Could you check a few things on this drawing? It's one solid part, dimensions in mm from its lowest x, y, z. A direction names the side the tool comes from. Give positions to 0.01 mm unless a question says otherwise; leave off trailing zeros. Loops run counter-clockwise (first coordinate to the right, second up) from the corner with the lowest first, then second, coordinate; pieces in that order, holes last. Notation, with made-up numbers: (85, 32.5) - (140, 32.5) arc R24 cw to (140, 58.5) - close; hole circle Ø6 at (74, 83). An arc over 180 degrees is marked (long way). Answer as a JSON object with one key per item and string values.
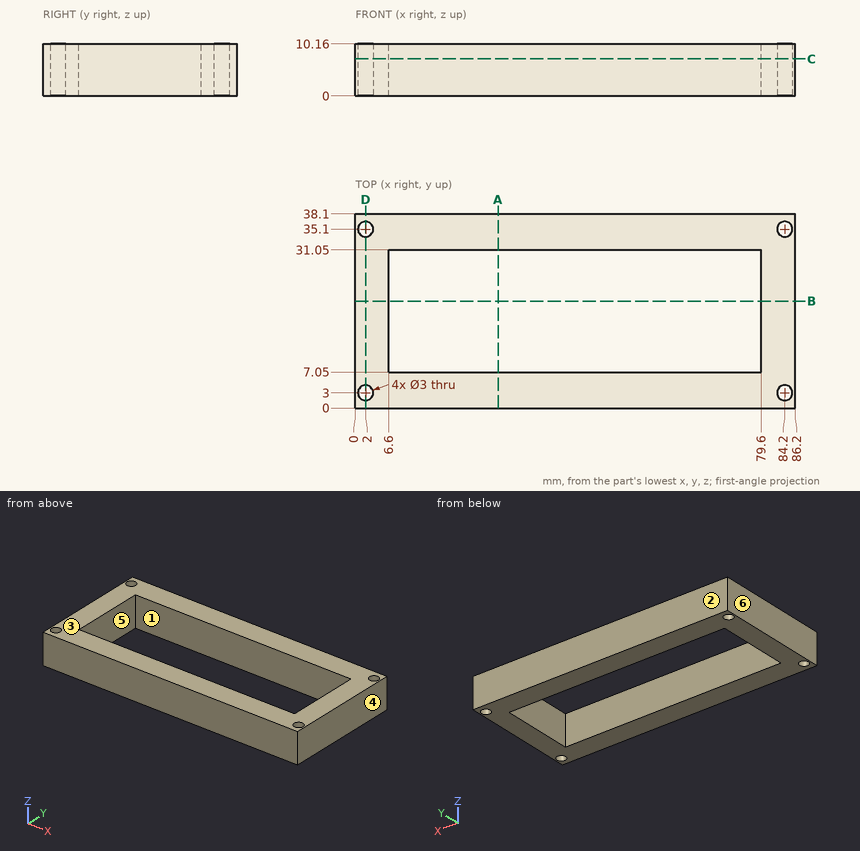
1) If we mould it in two halves opening along X, with no side actions, what happens to the marked faces 3, 4, 5 and 6? For each: released by +X, released by -X, zero draft, split by the parting line, or undercut.
Check sheet entries:
{"face 3": "zero draft", "face 4": "released by +X", "face 5": "undercut", "face 6": "released by -X"}
2) Imagine slicing it at D-D on x = 2. Write out the boundary of the cut face in (y, z), and give its area (3 significant figures).
Check sheet entries:
{"outline": "(0, 0) - (1.5, 0) - (1.5, 10.16) - (0, 10.16) - close; (4.5, 0) - (33.6, 0) - (33.6, 10.16) - (4.5, 10.16) - close; (36.6, 0) - (38.1, 0) - (38.1, 10.16) - (36.6, 10.16) - close", "area": "326 mm2"}
3) Imagine slicing it at A-A on x = 28. Write out the boundary of the cut face in (y, z).
Check sheet entries:
{"outline": "(0, 0) - (7.05, 0) - (7.05, 10.16) - (0, 10.16) - close; (31.05, 0) - (38.1, 0) - (38.1, 10.16) - (31.05, 10.16) - close"}
4) I'm going to push a flat-ended pin straight in: P1, Ø8, axis at x = 40.5, y = 6, coming from the -Z side. Where does the tip first touch, or does it pass through?
Check sheet entries:
{"P1": "z = 0"}
5) Imagine slicing it at B-B on y = 21. Write out the boundary of the cut face in (x, z), and give its area (3 significant figures).
Check sheet entries:
{"outline": "(0, 0) - (6.6, 0) - (6.6, 10.16) - (0, 10.16) - close; (79.6, 0) - (86.2, 0) - (86.2, 10.16) - (79.6, 10.16) - close", "area": "134 mm2"}
6) Which directions (+Z, -Z, +X, -X, +Y, -Y) give clear straight access to the entire face, cutting with the end or side of a thin tool? Please do the marked faces 1 and 2.
Check sheet entries:
{"face 1": "+Z, -Z", "face 2": "+Z, -Z, +X, -X, +Y"}
7) I need wall thicknesses on L1, parallel to Y at x = 84.2, z = 2.25; L2, parallel to X at y = 29, z = 7; L3, parallel to Y at x = 68, z = 6.75. Which ranges of each line are inside material? Lowest first, please.
Check sheet entries:
{"L1": "0 to 1.5, 4.5 to 33.6, 36.6 to 38.1", "L2": "0 to 6.6, 79.6 to 86.2", "L3": "0 to 7.05, 31.05 to 38.1"}
8) Imagine slicing it at C-C on z = 7.25. Write out the boundary of the cut face in (x, y), and give its area (3 significant figures).
Check sheet entries:
{"outline": "(0, 0) - (86.2, 0) - (86.2, 38.1) - (0, 38.1) - close; hole circle Ø3 at (2, 3); hole circle Ø3 at (2, 35.1); hole (6.6, 7.05) - (79.6, 7.05) - (79.6, 31.05) - (6.6, 31.05) - close; hole circle Ø3 at (84.2, 3); hole circle Ø3 at (84.2, 35.1)", "area": "1,500 mm2"}
